from build123d import *

# Parameters (mm, degrees)
SKETCH1_W                = 228.6
SKETCH1_H                = 609.6
BOSS_EXTRUDE1_DEPTH      = 6.35
CUT_EXTRUDE1_DEPTH       = 6.35
CUT_EXTRUDE4_DEPTH       = 1
CUT_EXTRUDE4_DEPTH_BACK  = 7.35
CUT_EXTRUDE7_DEPTH       = 1
CUT_EXTRUDE7_DEPTH_BACK  = 7.35
CUT_EXTRUDE8_DEPTH       = 1
CUT_EXTRUDE8_DEPTH_BACK  = 7.35
CUT_EXTRUDE9_DEPTH       = 1
CUT_EXTRUDE9_DEPTH_BACK  = 7.35
CUT_EXTRUDE10_DEPTH      = 1
CUT_EXTRUDE10_DEPTH_BACK = 7.35
CUT_EXTRUDE11_DEPTH      = 1
CUT_EXTRUDE11_DEPTH_BACK = 7.35
CUT_EXTRUDE12_DEPTH      = 1
CUT_EXTRUDE12_DEPTH_BACK = 7.35


with BuildPart() as part:
    # Sketch1 → Boss-Extrude1 (new body)
    with BuildSketch(Plane.XY):
        with Locations((-114.3, 304.8)):
            Rectangle(SKETCH1_W, SKETCH1_H)
    extrude(amount=BOSS_EXTRUDE1_DEPTH)

    # Sketch2 → Cut-Extrude1 (cut)
    with BuildSketch(Plane.XY.offset(6.35)):
        with BuildLine():
            Line((-165.095373919, 23.135327723), (-190.495373919, 23.135327723))
            ThreePointArc((-190.495373919, 23.135327723), (-196.845373919, 29.485327723), (-190.495373919, 35.835327723))
            Line((-190.495373919, 35.835327723), (-165.095373919, 35.835327723))
            ThreePointArc((-165.095373919, 35.835327723), (-158.745373919, 29.485327723), (-165.095373919, 23.135327723))
        make_face()
    extrude(amount=-CUT_EXTRUDE1_DEPTH, mode=Mode.SUBTRACT)

    # Sketch6 → Cut-Extrude4 (cut, two sides)
    with BuildSketch(Plane.XY.offset(6.35)) as cut_extrude4_sk:
        Polygon((-19.05, -1299.222032855), (-19.05, 0), (-19.05, 127), (0, 127), (1299.222032855, 127), (3207.394059988, -1636.743484042), (1889.122027132, -3062.965516897), align=None)
    extrude(amount=CUT_EXTRUDE4_DEPTH, mode=Mode.SUBTRACT)
    extrude(cut_extrude4_sk.sketch, amount=-CUT_EXTRUDE4_DEPTH_BACK, mode=Mode.SUBTRACT)

    # Sketch5 → Cut-Extrude7 (cut, two sides)
    with BuildSketch(Plane.XY.offset(6.35)) as cut_extrude7_sk:
        Polygon((-19.05, 1908.822032855), (-19.05, 609.6), (-19.05, 482.6), (0, 482.6), (1299.222032855, 482.6), (3207.394059988, 2246.343484042), (1889.122027132, 3672.565516897), align=None)
    extrude(amount=CUT_EXTRUDE7_DEPTH, mode=Mode.SUBTRACT)
    extrude(cut_extrude7_sk.sketch, amount=-CUT_EXTRUDE7_DEPTH_BACK, mode=Mode.SUBTRACT)

    # Sketch11 → Cut-Extrude8 (cut, two sides)
    with BuildSketch(Plane.XY.offset(6.35)) as cut_extrude8_sk:
        Polygon((-12.7, 1549.984641462), (-12.7, 482.6), (-12.7, 127), (-12.7, -940.384641462), (2122.069282924, -940.384641462), (2122.069282924, 1549.984641462), align=None)
    extrude(amount=CUT_EXTRUDE8_DEPTH, mode=Mode.SUBTRACT)
    extrude(cut_extrude8_sk.sketch, amount=-CUT_EXTRUDE8_DEPTH_BACK, mode=Mode.SUBTRACT)

    # Sketch15 → Cut-Extrude9 (cut, two sides)
    with BuildSketch(Plane.XY.offset(6.35)) as cut_extrude9_sk:
        Polygon((-209.55, -1291.190200556), (-209.55, 0), (-209.55, 127), (-228.6, 127), (-1519.790200556, 127), (-3416.571079884, -1625.401447117), (-2106.330879328, -3043.591647673), align=None)
    extrude(amount=CUT_EXTRUDE9_DEPTH, mode=Mode.SUBTRACT)
    extrude(cut_extrude9_sk.sketch, amount=-CUT_EXTRUDE9_DEPTH_BACK, mode=Mode.SUBTRACT)

    # Sketch12 → Cut-Extrude10 (cut, two sides)
    with BuildSketch(Plane.XY.offset(6.35)) as cut_extrude10_sk:
        Polygon((-209.55, 1900.790200556), (-209.55, 609.6), (-209.55, 482.6), (-228.6, 482.6), (-1519.790200556, 482.6), (-3416.571079884, 2235.001447117), (-2106.330879328, 3653.191647673), align=None)
    extrude(amount=CUT_EXTRUDE10_DEPTH, mode=Mode.SUBTRACT)
    extrude(cut_extrude10_sk.sketch, amount=-CUT_EXTRUDE10_DEPTH_BACK, mode=Mode.SUBTRACT)

    # Sketch16 → Cut-Extrude11 (cut, two sides)
    with BuildSketch(Plane.XY.offset(6.35)) as cut_extrude11_sk:
        Polygon((-215.9, 1539.868828907), (-215.9, 482.6), (-215.9, 127), (-215.9, -930.268828907), (-2330.437657814, -930.268828907), (-2330.437657814, 1539.868828907), align=None)
    extrude(amount=CUT_EXTRUDE11_DEPTH, mode=Mode.SUBTRACT)
    extrude(cut_extrude11_sk.sketch, amount=-CUT_EXTRUDE11_DEPTH_BACK, mode=Mode.SUBTRACT)

    # Sketch18 → Cut-Extrude12 (cut, two sides)
    with BuildSketch(Plane.XY.offset(6.35)) as cut_extrude12_sk:
        Polygon((-82.55, -1258.029458787), (-82.55, 0), (-82.55, 6.35), (-146.05, 6.35), (-146.05, 0), (-146.05, -1258.029458787), (-146.05, -3774.088376361), (-82.55, -3774.088376361), align=None)
    extrude(amount=CUT_EXTRUDE12_DEPTH, mode=Mode.SUBTRACT)
    extrude(cut_extrude12_sk.sketch, amount=-CUT_EXTRUDE12_DEPTH_BACK, mode=Mode.SUBTRACT)


solid = part.part
The listing builds one solid part. Answer for the finished solid, in the listing's coordinates (mm). Round coordinates to 2 decimals unless told otherwise and drop trailing zeros. Write each loop counter-clockwise with the first axis right and the second up, starting at its lowest first coordinate (ties: lowest second). Pieces come first, ordered by that corner, then holes. Notation, with made-up numbers: M 22.5,47.5 L 42.5,47.5 A27 cw 42.5,80.5 Z; hole C -37,-19 d7. An arc over 180 degrees is marked long. Write each question's results on one line, items separated by ' | '. Start each with the question number.
Item 1: Flat-ended cylindrical pins translate along their axes: pin 1 Ø1.9 at (y, z) = (559.5, 3.5) entering from -X; pin 2 Ø1.9 at (x, z) = (-14.5, 2) entering from +Y; pin 3 Ø1 at (y, z) = (526, 5) entering from +X. Find the tip coordinate at first contact, or state that the pin passes through.
Item 2: A cutting plane is placed at B-B on y = 515.5. Write down the section's boundary in (x, z).
Item 3: A cutting plane is placed at A-A on z = 2. Write down the section's boundary in (x, y), and give its area (3 significant figures).
Item 4: Straight lines are drawn through the part: L1, parallel to Y at x = -172, z = 3.5; L2, parallel to X at y = 504, z = 5.75; L3, parallel to Y at x = -141.5, z = 1.5. For each, find the intervals that lie inside material, in ascending order. Write a range as [from, to].
Check sheet entries:
1) pin 1: x = -209.55 | pin 2: y = 482.6 | pin 3: x = -19.05
2) outline: M -209.55,0 L -19.05,0 L -19.05,6.35 L -209.55,6.35 Z
3) outline: M -215.9,127 L -209.55,127 L -209.55,0 L -146.05,0 L -146.05,6.35 L -82.55,6.35 L -82.55,0 L -19.05,0 L -19.05,127 L -12.7,127 L -12.7,482.6 L -19.05,482.6 L -19.05,609.6 L -209.55,609.6 L -209.55,482.6 L -215.9,482.6 Z; hole M -190.5,23.14 L -165.1,23.14 A6.35 ccw -165.1,35.84 L -190.5,35.84 A6.35 ccw Z | area: 120,000 mm²
4) L1: [0, 23.14], [35.84, 609.6] | L2: [-209.55, -19.05] | L3: [6.35, 609.6]
